Work out the finished part from the listing and answer in its coordinate system (mm). A direction names the side the tool comes from. Round coordinates to 2 decimals unless told otherwise and drop trailing zeros. Order: outer loops, then holes, each group sorted by start corner. A loop starts at its lowest first (then second) coordinate and runs counter-clockwise, first axis right, second up. Notation, with made-up numbers: M 70.5,-30 L 92.5,-30 A32 ccw 92.5,7 Z; hole C 22.5,36 d7. An arc over 180 degrees is marked long. Answer as a JSON object with one key per item and string values. Group by question number.
from build123d import *

# Parameters (mm, degrees)
BOSS_EXTRUDE1_DEPTH = 5


with BuildPart() as part:
    # Sketch2 → Boss-Extrude1 (new body)
    with BuildSketch(Plane.XY):
        with BuildLine():
            Line((0, 3), (49.5, 3))
            ThreePointArc((49.5, 3), (52.5, 0), (49.5, -3))
            Line((49.5, -3), (3, -3))
            Line((3, -3), (-6.616826065, -3))
            Line((-6.616826065, -3), (-6.616826065, 3))
            Line((-6.616826065, 3), (0, 3))
        make_face()
        with BuildLine():
            Line((0, -1.5), (49.5, -1.5))
            ThreePointArc((49.5, -1.5), (51, 0), (49.5, 1.5))
            Line((49.5, 1.5), (0, 1.5))
            ThreePointArc((0, 1.5), (-1.5, 0), (0, -1.5))
        make_face(mode=Mode.SUBTRACT)
    extrude(amount=BOSS_EXTRUDE1_DEPTH)


solid = part.part
Item 1: Consider L1, parallel to Y at x = 48, z = 2.2; L2, parallel to X at y = 0.1, z = 2.2; L3, parallel to X at y = 1.2, z = 1.5. Determine where each line is inside the solid, lowest interval first.
Item 2: The mould has two halves that part along X. Classify faces 1 (the cylindrical face through (52.5, 0.1, 2.5)), 2 (the flat face through (22, -3, 2)), 3 (the flat face through (25, 1.5, 2)): +X half, -X half, draft (parallel to the pull), parting line (faces both ways), or undercut.
Item 3: Find section B-B (x = -0.5). Give the vertices of the cut face in (y, z), and give its area (3 significant figures).
Item 4: Find section C-C (z = 0.9). Give the vertices of the cut face in (x, y), and give its area (3 significant figures).
Item 5: This flat-tipped pin is pushed along its axis until it touches: pin 1 (2 mm diameter, centred on x = 43.5, y = 1, fed in from -Z). Where does it stop, or does it pass through?
Item 6: A tool of negligible diameter and unlimited length cuts with its end or side. For faces 4 (the flat face through (-6.617, 0, 2)), 5 (the cylindrical face through (-1.5, 0, 2.5)), from which of +Z, -Z, +X, -X, +Y, -Y can it reach the whole face along a straight path? Write none if from no direction.
Item 7: Find section A-A (y = 0). Give the vertices of the cut face in (x, z).
Responses:
{
 "1": {"L1": "y = -3 to -1.5, 1.5 to 3", "L2": "x = -6.62 to -1.5, 51 to 52.5", "L3": "x = -6.62 to -0.9, 50.4 to 52.25"},
 "2": {"face 1": "+X half", "face 2": "draft", "face 3": "undercut"},
 "3": {"outline": "M -3,0 L -1.41,0 L -1.41,5 L -3,5 Z; M 1.41,0 L 3,0 L 3,5 L 1.41,5 Z", "area": "15.9 mm^2"},
 "4": {"outline": "M -6.62,-3 L 49.5,-3 A3 ccw 49.5,3 L -6.62,3 Z; hole M 0,-1.5 L 49.5,-1.5 A1.5 ccw 49.5,1.5 L 0,1.5 A1.5 ccw Z", "area": "195 mm^2"},
 "5": {"pin 1": "stops at z = 0"},
 "6": {"face 4": "+Z, -Z, -X, +Y, -Y", "face 5": "+Z, -Z"},
 "7": {"outline": "M -6.62,0 L -1.5,0 L -1.5,5 L -6.62,5 Z; M 51,0 L 52.5,0 L 52.5,5 L 51,5 Z"}
}
